Check sheet for the modelled part. Datum: model origin and axes. Units: mm. Face numbers are marked on the shaded views. A direction names the side the tool comes from. Coordinates: 2 decimals unless noted, no trailing zeros. Loops run counter-clockwise (first coordinate to the right, second up) from the corner with the lowest first, then second, coordinate; pieces in that order, holes last. Notation, with made-up numbers: (-36.75, 6) - (5.25, 6) arc R37 cw to (5.25, 42) - close; hole circle Ø1 at (-4.75, -21.5). An arc over 180 degrees is marked (long way). Use a Markdown table: item, result. Add a question column.
1) Sectioned sample at C-C, the plane x = -14.25. State how many separate pieces and enclosed holes the cut face has, then the cut area to 3 significant figures.
2) Draft check along Y on the marked faces 1, 2, 3 and 4. Enter one of: pulls with the +Y half, pulls with the -Y half, needs draft (parallel to the pull), parting line crosses it, or undercut.
3) Thickness scan on line 1 (Z direction, x = -4.5, y = 50); line 2 (Y direction, x = -10.5, z = 9.5); line 3 (Y direction, x = -0.75, z = 32). Record the ranges inside material, lowest first.
4) Sectioned sample at D-D, the plane y = 30. Enter the section's corners in (x, z).
5) Sectioned sample at A-A, the plane y = 45.5. Enter the section's corners in (x, z), then the cut area to 3 significant figures.
6) Tool access check on the marked faces 5, 6, 7, 8 and 9. Record the directions out of +Z, -Z, +X, -X, +Y, -Y that give a thin tool (end or side, any length) a straight path to the whole face; none if there is none.
7) Go/stop test with flat-tipped pins: P1, Ø5, axis at x = -15, y = 6, coming from the -Z side; P2, Ø3.5, axis at y = 61, z = 40.5, coming from the -X side; P3, Ø2, axis at y = 58.5, z = 30, coming from the +X side; P4, Ø5.5, axis at x = -5, z = 54.5, coming from the -Y side. Record where each tip stops, or that it passes through.
8) Sectioned sample at B-B, the plane z = 54.5. Enter the section's corners in (x, y).
from build123d import *

# Parameters (mm, degrees)
SKETCH1_W           = 20
SKETCH1_H           = 50
BOSS_EXTRUDE1_DEPTH = 70
SKETCH2_R           = 2
SKETCH2_R_2         = 11.5
CUT_EXTRUDE2_DEPTH  = 60
SKETCH4_W           = 25
SKETCH4_H           = 12
CUT_EXTRUDE3_DEPTH  = 60
SKETCH8_R           = 2
CUT_EXTRUDE5_DEPTH  = 15
SKETCH9_W           = 42
SKETCH9_H           = 42
CUT_EXTRUDE6_DEPTH  = 6
CUT_EXTRUDE8_DEPTH  = 30
SKETCH12_W          = 20
SKETCH12_H          = 5
BOSS_EXTRUDE2_DEPTH = 9
BOSS_EXTRUDE3_DEPTH = 20
SKETCH15_R          = 2
CUT_EXTRUDE9_DEPTH  = 10
SKETCH18_R          = 3.5
CUT_EXTRUDE12_DEPTH = 53
SKETCH17_R          = 3.5
CUT_EXTRUDE13_DEPTH = 16
SKETCH19_R          = 2
CUT_EXTRUDE14_DEPTH = 25


with BuildPart() as part:
    # Sketch1 → Boss-Extrude1 (new body)
    with BuildSketch(Plane(origin=(0, 0, 0), x_dir=(1, 0, 0), z_dir=(0, 1, 0))):
        with Locations((-10, -25)):
            Rectangle(SKETCH1_W, SKETCH1_H)
    extrude(amount=BOSS_EXTRUDE1_DEPTH)

    # Sketch2 → Cut-Extrude2 (cut)
    with BuildSketch(Plane(origin=(0, 0, 0), x_dir=(0, 0, -1), z_dir=(1, 0, 0))):
        with Locations((-9.5, 61)):
            Circle(SKETCH2_R)
        with Locations((-25, 45.5)):
            Circle(SKETCH2_R_2)
        with Locations((-9.5, 30)):
            Circle(SKETCH2_R)
        with Locations((-40.5, 30)):
            Circle(SKETCH2_R)
        with Locations((-40.5, 61)):
            Circle(SKETCH2_R)
    extrude(amount=-CUT_EXTRUDE2_DEPTH, mode=Mode.SUBTRACT)

    # Sketch4 → Cut-Extrude3 (cut)
    with BuildSketch(Plane(origin=(0, 0, 0), x_dir=(0, 0, -1), z_dir=(1, 0, 0))):
        with Locations((-37.5, 6)):
            Rectangle(SKETCH4_W, SKETCH4_H)
    extrude(amount=-CUT_EXTRUDE3_DEPTH, mode=Mode.SUBTRACT)

    # Sketch8 → Cut-Extrude5 (cut)
    with BuildSketch(Plane(origin=(0, 0, 0), x_dir=(-1, 0, 0), z_dir=(0, 0, -1))):
        with Locations((15, 6)):
            Circle(SKETCH8_R)
        with Locations((5, 6)):
            Circle(SKETCH8_R)
    extrude(amount=-CUT_EXTRUDE5_DEPTH, mode=Mode.SUBTRACT)

    # Sketch9 → Cut-Extrude6 (cut)
    with BuildSketch(Plane(origin=(0, 0, 0), x_dir=(0, 0, -1), z_dir=(1, 0, 0))):
        with Locations((-25, 45.5)):
            Rectangle(SKETCH9_W, SKETCH9_H)
    extrude(amount=-CUT_EXTRUDE6_DEPTH, mode=Mode.SUBTRACT)

    # Sketch11 → Cut-Extrude8 (cut)
    with BuildSketch(Plane(origin=(0, 0, 0), x_dir=(0, 0, -1), z_dir=(1, 0, 0))):
        Polygon((-19, 0), (0, 0), (0, 12), align=None)
    extrude(amount=-CUT_EXTRUDE8_DEPTH, mode=Mode.SUBTRACT)

    # Sketch12 → Boss-Extrude2 (add)
    with BuildSketch(Plane.XY.offset(50)):
        with Locations((-10, 14.5)):
            Rectangle(SKETCH12_W, SKETCH12_H)
    extrude(amount=BOSS_EXTRUDE2_DEPTH)

    # Sketch14 → Boss-Extrude3 (add)
    with BuildSketch(Plane(origin=(0, 0, 0), x_dir=(0, 0, -1), z_dir=(1, 0, 0))):
        Polygon((-50, 17), (-59, 17), (-50, 22), align=None)
    extrude(amount=-BOSS_EXTRUDE3_DEPTH)

    # Sketch15 → Cut-Extrude9 (cut)
    with BuildSketch(Plane(origin=(0, 12, 0), x_dir=(-1, 0, 0), z_dir=(0, -1, 0))):
        with Locations(Location((5, -54.5, 0), (0, 0, 90))):
            Circle(SKETCH15_R)
        with Locations(Location((15, -54.5, 0), (0, 0, 90))):
            Circle(SKETCH15_R)
    extrude(amount=-CUT_EXTRUDE9_DEPTH, mode=Mode.SUBTRACT)

    # Sketch18 → Cut-Extrude12 (cut)
    with BuildSketch(Plane(origin=(0, 70, 0), x_dir=(1, 0, 0), z_dir=(0, 1, 0))):
        with Locations(Location((-15, -54.5, 0), (0, 0, 270))):
            Circle(SKETCH18_R)
        with Locations(Location((-5, -54.5, 0), (0, 0, 270))):
            Circle(SKETCH18_R)
    extrude(amount=-CUT_EXTRUDE12_DEPTH, mode=Mode.SUBTRACT)

    # Sketch17 → Cut-Extrude13 (cut)
    with BuildSketch(Plane(origin=(0, 0, 0), x_dir=(-1, 0, 0), z_dir=(0, 0, -1))):
        with Locations((15, 6)):
            Circle(SKETCH17_R)
        with Locations((5, 6)):
            Circle(SKETCH17_R)
    extrude(amount=-CUT_EXTRUDE13_DEPTH, mode=Mode.SUBTRACT)

    # Sketch19 → Cut-Extrude14 (cut)
    with BuildSketch(Plane(origin=(0, 0, 16), x_dir=(-1, 0, 0), z_dir=(0, 0, -1))):
        with Locations((5, 6)):
            Circle(SKETCH19_R)
        with Locations((15, 6)):
            Circle(SKETCH19_R)
    extrude(amount=-CUT_EXTRUDE14_DEPTH, mode=Mode.SUBTRACT)


solid = part.part
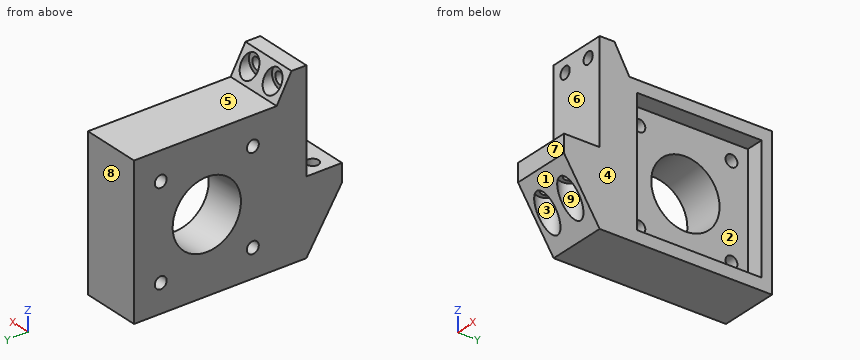
Solved:
| question | item | result |
|---|---|---|
| 1 | separate pieces | 3 |
| 1 | enclosed holes | 5 |
| 1 | area | 2,570 mm2 |
| 2 | face 1 | pulls with the -Y half |
| 2 | face 2 | undercut |
| 2 | face 3 | undercut |
| 2 | face 4 | needs draft |
| 3 | line 1 | z = 0 to 4, 46 to 50 |
| 3 | line 2 | y = 6 to 28, 32 to 59, 63 to 70 |
| 3 | line 3 | y = 12 to 24.5, 66.5 to 70 |
| 4 | outline | (-20, 0) - (0, 0) - (0, 4) - (-6, 4) - (-6, 7.5) - (-20, 7.5) - close; (-20, 11.5) - (-6, 11.5) - (-6, 38.5) - (-20, 38.5) - close; (-20, 42.5) - (-6, 42.5) - (-6, 46) - (0, 46) - (0, 50) - (-20, 50) - close |
| 5 | outline | (-20, 0) - (0, 0) - (0, 4) - (-6, 4) - (-6, 13.5) - (-20, 13.5) - close; (-20, 36.5) - (-6, 36.5) - (-6, 46) - (0, 46) - (0, 50) - (-20, 50) - close |
| 5 | area | 426 mm2 |
| 6 | face 5 | +Z, +X, -X, +Y |
| 6 | face 6 | +Z, +X, -X, -Y |
| 6 | face 7 | +Z, -Z, +X, -X, -Y |
| 6 | face 8 | +Z, -Z, +X, -X, +Y |
| 6 | face 9 | -Z |
| 7 | P1 | stops at z = 16 |
| 7 | P2 | passes through |
| 7 | P3 | stops at x = -6 |
| 7 | P4 | stops at y = 12 |
| 8 | outline | (-20, 12) - (-17, 12) - (-17, 17) - (-18.5, 17) - (-18.5, 19.5) - (-20, 19.5) - close; (-13, 12) - (-7, 12) - (-7, 17) - (-8.5, 17) - (-8.5, 19.5) - (-11.5, 19.5) - (-11.5, 17) - (-13, 17) - close; (-3, 12) - (0, 12) - (0, 19.5) - (-1.5, 19.5) - (-1.5, 17) - (-3, 17) - close |
